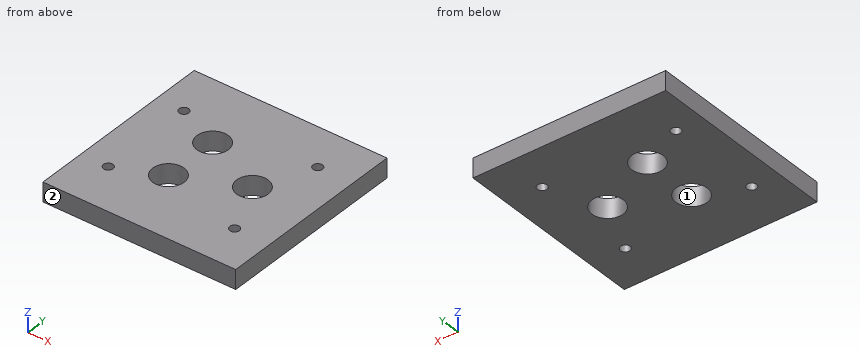
```python
from build123d import *

# Parameters (mm, degrees)
F0_W     = 20
F0_H     = 20
F0_R     = 1.63
F1_DEPTH = 2
F3_D     = 1


with BuildPart() as f1:
    # F0 (on Top) → F1 (new body)
    with BuildSketch(Plane.XY):
        Rectangle(F0_W, F0_H)
        with Locations((-2.54, -2.92)):
            Circle(F0_R, mode=Mode.SUBTRACT)
        with Locations((-2.54, 2.92)):
            Circle(F0_R, mode=Mode.SUBTRACT)
        with Locations((3.88, 0)):
            Circle(F0_R, mode=Mode.SUBTRACT)
    extrude(amount=F1_DEPTH)

    # F3 (through all)
    with Locations(Plane.XY.offset(2)):
        with Locations((6.35, 5.5), (6.35, -5.5), (-7.15, -5), (-7.15, 5)):
            Hole(F3_D / 2)


solid = f1.part
```
Can you work these out from the model? Positions are in its coordinate system, mm. Face numbers are marked on the shaded views. Give positions to 0.01 mm unless a question says otherwise; leave off trailing zeros. Write each loop counter-clockwise with the first axis right and the second up, starting at its lowest first coordinate (ties: lowest second). Pieces come first, ordered by that corner, then holes. Notation, with made-up numbers: (32.5, 29) - (54.5, 29) arc R11 cw to (54.5, 48) - close; hole circle Ø6 at (-6, 79). An arc over 180 degrees is marked (long way). Write item = value, one per line. Start each with the question number.
1. Please list where these lines run through material, in increasing order: line 1 (Y direction, x = -2.54, z = 1.55); line 2 (Y direction, x = 6.35, z = 1.3); line 3 (Y direction, x = 3.75, z = 1.9).
2. Imagine slicing it at B-B (y = -2.92). Please give me the cut outline in (x, z), and give its area (3 significant figures).
3. Imagine slicing it at A-A (x = 6.35). Please give me the cut outline in (y, z).
4. Imagine slicing it at C-C (z = 0.7). Please give me the cut outline in (x, y).
5. Thinking about a two-plate mould opening in X: for the marked faces 1 and 2, which applies, released by +X, released by -X, zero draft, split by the parting line, or undercut?
6. Imagine slicing it at D-D (x = 3.88). Please give me the cut outline in (y, z), and give its area (3 significant figures).
Worked answers:
q1.line_1 = -10 to -4.55, -1.29 to 1.29, 4.55 to 10
q1.line_2 = -10 to -6, -5 to 5, 6 to 10
q1.line_3 = -10 to -1.62, 1.62 to 10
q2.outline = (-10, 0) - (-4.17, 0) - (-4.17, 2) - (-10, 2) - close; (-0.91, 0) - (10, 0) - (10, 2) - (-0.91, 2) - close
q2.area = 33.5 mm2
q3.outline = (-10, 0) - (-6, 0) - (-6, 2) - (-10, 2) - close; (-5, 0) - (5, 0) - (5, 2) - (-5, 2) - close; (6, 0) - (10, 0) - (10, 2) - (6, 2) - close
q4.outline = (-10, -10) - (10, -10) - (10, 10) - (-10, 10) - close; hole circle Ø1 at (-7.15, -5); hole circle Ø1 at (-7.15, 5); hole circle Ø3.26 at (-2.54, -2.92); hole circle Ø3.26 at (-2.54, 2.92); hole circle Ø3.26 at (3.88, 0); hole circle Ø1 at (6.35, -5.5); hole circle Ø1 at (6.35, 5.5)
q5.face_1 = undercut
q5.face_2 = zero draft
q6.outline = (-10, 0) - (-1.63, 0) - (-1.63, 2) - (-10, 2) - close; (1.63, 0) - (10, 0) - (10, 2) - (1.63, 2) - close
q6.area = 33.5 mm2
